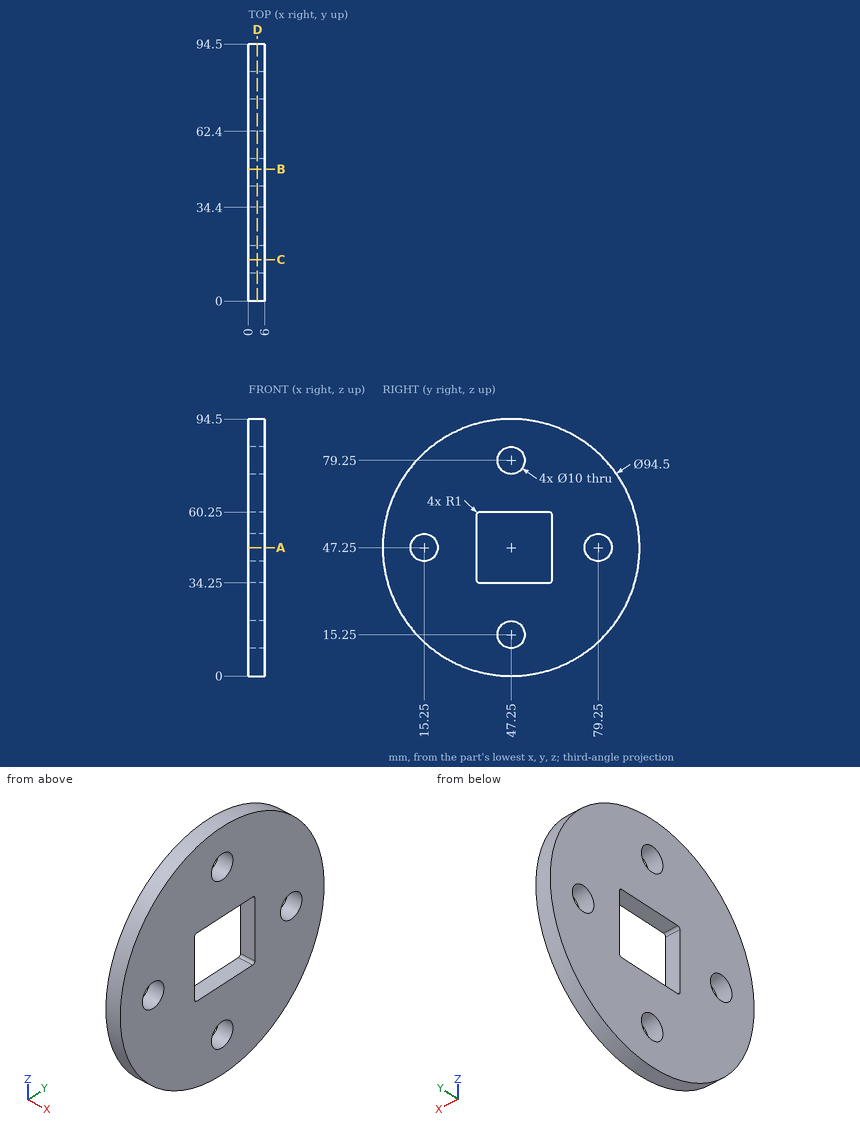
Could you check a few things on this drawing? It's one solid part, dimensions in mm from its lowest x, y, z. Coordinates: 2 decimals unless noted, no trailing zeros. Write each loop counter-clockwise with the first axis right and the second up, starting at its lowest first coordinate (ties: lowest second). Pieces come first, ordered by that corner, then holes. Notation, with made-up numbers: M -39.5,58.5 L -19.5,58.5 A15 cw -19.5,80.5 Z; hole C 12,53.25 d3. An arc over 180 degrees is marked long. One line per question, with ' | ' between items.
1) Imagine slicing it at D-D, the plane x = 3.35. Write out the boundary of the cut face in (y, z).
Checks:
outline: C 47.25,47.25 d94.5; hole C 15.25,47.25 d10; hole M 34.4,35.25 A1 ccw 35.4,34.25 L 61.4,34.25 A1 ccw 62.4,35.25 L 62.4,59.25 A1 ccw 61.4,60.25 L 35.4,60.25 A1 ccw 34.4,59.25 Z; hole C 47.25,15.25 d10; hole C 47.25,79.25 d10; hole C 79.25,47.25 d10
2) For pin 1 Ø1.5 at (y, z) = (34.5, 42.5) entering from -X; pin 2 Ø3 at (x, z) = (5.5, 61) entering from +Y; pin 3 Ø1 at (x, y) = (4.5, 26) entering from -Z; pin 4 Ø3 at (x, y) = (2.5, 52) entering from +Z, each with a flat end and sliding along its axis, tell me the tip position at first contact or that it passes through.
Checks:
pin 1: x = 0 | pin 2: y = 92.88 | pin 3: z = 4.8 | pin 4: z = 94.39
3) Imagine slicing it at A-A, the plane z = 47.25. Write out the boundary of the cut face in (x, y), and give its area (3 significant figures).
Checks:
outline: M 0,0 L 6,0 L 6,10.25 L 0,10.25 Z; M 0,20.25 L 6,20.25 L 6,34.4 L 0,34.4 Z; M 0,62.4 L 6,62.4 L 6,74.25 L 0,74.25 Z; M 0,84.25 L 6,84.25 L 6,94.5 L 0,94.5 Z | area: 279 mm²
4) Imagine slicing it at B-B, the plane y = 48.5. Write out the boundary of the cut face in (x, z), and give its area (3 significant figures).
Checks:
outline: M 0,0.02 L 6,0.02 L 6,10.41 L 0,10.41 Z; M 0,20.09 L 6,20.09 L 6,34.25 L 0,34.25 Z; M 0,60.25 L 6,60.25 L 6,74.41 L 0,74.41 Z; M 0,84.09 L 6,84.09 L 6,94.48 L 0,94.48 Z | area: 295 mm²
5) I need wall thicknesses on probe 1 along Y at (x, z) = (4.4, 47.25); probe 2 along Y at (x, z) = (2.6, 36); probe 3 along Z at (x, y) = (1.4, 80). Which ranges of each line are inside material? Lowest first, please. Write a range as [from, to].
Checks:
probe 1: [0, 10.25], [20.25, 34.4], [62.4, 74.25], [84.25, 94.5] | probe 2: [1.36, 34.4], [62.4, 93.14] | probe 3: [13.19, 42.31], [52.19, 81.31]
6) Imagine slicing it at C-C, the plane y = 15.25. Write out the boundary of the cut face in (x, z).
Checks:
outline: M 0,12.49 L 6,12.49 L 6,42.25 L 0,42.25 Z; M 0,52.25 L 6,52.25 L 6,82.01 L 0,82.01 Z
